Print and shaded views of the part. All mm, measured from the part's lowest x, y and z. Coordinates: 2 decimals unless noted, no trailing zeros. Order: outer loops, then holes, each group sorted by start corner. A loop starts at its lowest first (then second) coordinate and runs counter-clockwise, first axis right, second up. Notation, with made-up numbers: M -6.75,36.25 L 19.25,36.25 A19 ccw 19.25,58.25 Z; hole C 25,68.5 d7. An arc over 180 degrees is marked long. Return JSON: item names as keys, results as strings.
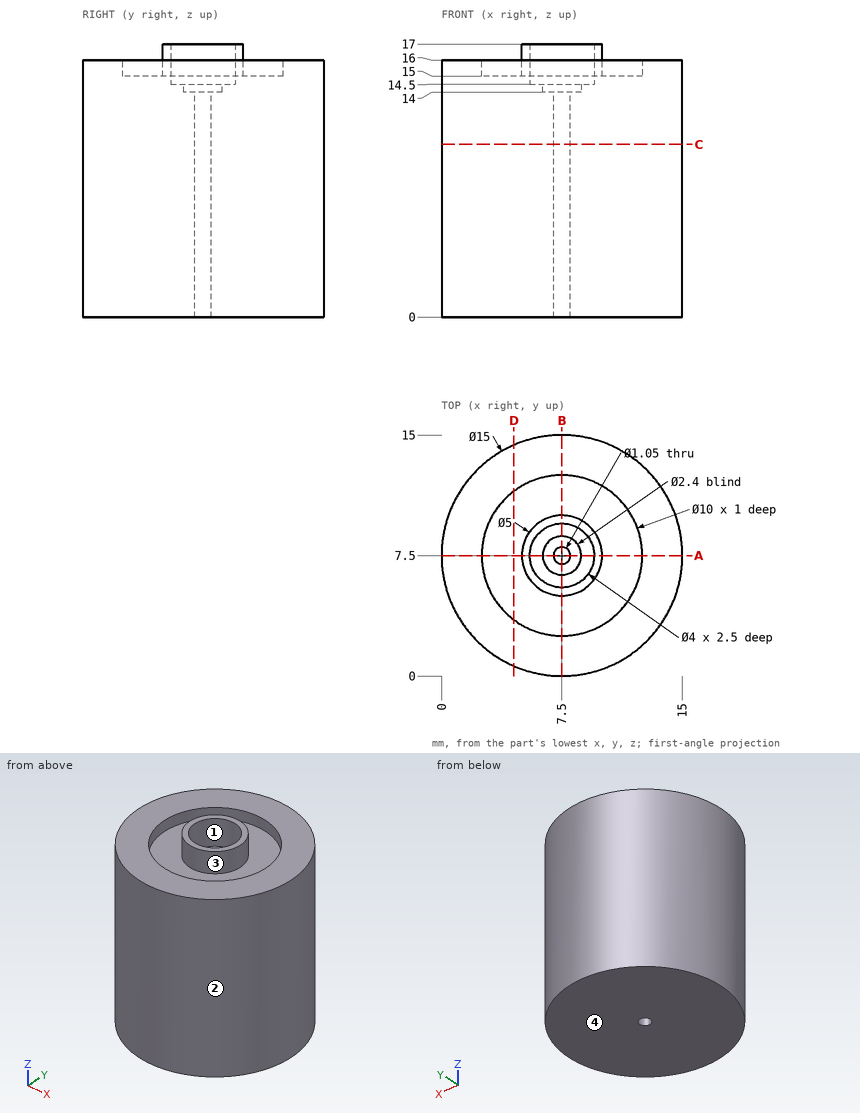
Item 1: Saw through at A-A (y = 7.5). Write the cut outline in (x, z) (3 decimals).
Check result:
{"outline": "M 0,0 L 6.975,0 L 6.975,14 L 6.3,14 L 6.3,14.5 L 5.5,14.5 L 5.5,17 L 5,17 L 5,15 L 2.5,15 L 2.5,16 L 0,16 Z; M 8.025,0 L 15,0 L 15,16 L 12.5,16 L 12.5,15 L 10,15 L 10,17 L 9.5,17 L 9.5,14.5 L 8.7,14.5 L 8.7,14 L 8.025,14 Z"}
Item 2: Saw through at D-D (x = 4.5). Write the cut outline in (y, z), and give its area (3 significant figures).
Check result:
{"outline": "M 0.63,0 L 14.37,0 L 14.37,16 L 11.5,16 L 11.5,15 L 3.5,15 L 3.5,16 L 0.63,16 Z", "area": "212 mm2"}
Item 3: Drop flat-ended pins along their axis: pin 1 Ø1 at (y, z) = (4.5, 7.5) entering from -X; pin 2 Ø2 at (x, y) = (8, 7) entering from +Z; pin 3 Ø8 at (x, y) = (1.5, 2.5) entering from +Z. Give the stop position or say it passes through.
Check result:
{"pin 1": "stops at x = 0.43", "pin 2": "stops at z = 14.5", "pin 3": "stops at z = 16"}
Item 4: Saw through at C-C (z = 10.75). Write the cut outline in (x, y) (3 decimals).
Check result:
{"outline": "C 7.5,7.5 d15; hole C 7.5,7.5 d1.05"}
Item 5: Wall check: line 1 (Y direction, x = 7.5, z = 15.55); line 2 (Y direction, x = 7.5, z = 5.5) (3 decimals); line 3 (Y direction, x = 7.5, z = 14.4). Give the ranges that are in metal, low to high.
Check result:
{"line 1": "y = 0 to 2.5, 5 to 5.5, 9.5 to 10, 12.5 to 15", "line 2": "y = 0 to 6.975, 8.025 to 15", "line 3": "y = 0 to 6.3, 8.7 to 15"}
Item 6: Pull direction X, two halves, no side cores. Call the marked faces 1, 2, 3 and 4: +X half, -X half, draft (parallel to the pull), parting line (faces both ways), or undercut.
Check result:
{"face 1": "undercut", "face 2": "parting line", "face 3": "undercut", "face 4": "draft"}
